The listing builds one solid part. Answer for the finished solid, in the listing's coordinates (mm). A direction names the side the tool comes from. Coordinates: 2 decimals unless noted, no trailing zeros. Order: outer loops, then holes, each group sorted by start corner. A loop starts at its lowest first (then second) coordinate and runs counter-clockwise, first axis right, second up. Notation, with made-up numbers: (78, 13.5) -> (125, 13.5) arc R22 ccw to (125, 26.5) -> close; hole circle Ø4 at (73, 11.25). An arc over 180 degrees is marked (long way). Answer in a Markdown table with one row per item.
```python
from build123d import *

# Parameters (mm, degrees)
F0_R     = 58.419928
F0_R_2   = 50.653175
F4_DEPTH = 8.255


with BuildPart() as f3:
    # F1 (on Right) → F3 (revolve)
    with BuildSketch(Plane.YZ):
        with BuildLine():
            Line((-9.656509, 58.766587), (9.687974, 58.134703))
            ThreePointArc((9.687974, 58.134703), (0.316333, 67.653236), (-9.656509, 58.766587))
        make_face()
    revolve(axis=Axis((0, -0.11386, 0), (0, -1, 0)))

    # F0 (on Front) → F4 (join, symmetric)
    with BuildSketch(Plane.XZ):
        Circle(F0_R)
        Circle(F0_R_2, mode=Mode.SUBTRACT)
    extrude(amount=F4_DEPTH, both=True)


solid = f3.part
```
(1) Find the intervals of material crossed by line 1 along X through (y, z) = (-5, -23); line 2 along Z through (x, y) = (52.5, -4); line 3 along X through (y, z) = (-6, 21.5), in increasing order. Write a range as from..to.
Check values:
| item | result |
|---|---|
| line 1 | -62.15..-53.91, -53.7..-45.13, 45.13..53.7, 53.91..62.15 |
| line 2 | -41.29..-25.99, -25.62..25.62, 25.99..41.29 |
| line 3 | -61.95..-54.56, -54.32..-45.86, 45.86..54.32, 54.56..61.95 |
(2) A cutting plane is placed at C-C, the plane y = 2.5. Determine the outline of the cut face in (x, z), then the cut area to 3 significant figures.
Check values:
| item | result |
|---|---|
| outline | circle Ø134.66 at (0, 0); hole circle Ø101.31 at (0, 0) |
| area | 6,180 mm² |
(3) Flat-ended cylindrical pins translate along their axes: pin 1 (5 mm diameter, centred on x = -50, y = -4.5, fed in from +Z); pin 2 (2 mm diameter, centred on y = -0.5, z = 16, fed in from +X); pin 3 (5 mm diameter, centred on y = 0, z = 45, fed in from +X). Find the tip coordinate at first contact, or state that the pin passes through.
Check values:
| item | result |
|---|---|
| pin 1 | z = 47.06 |
| pin 2 | x = 65.97 |
| pin 3 | x = 52.64 |
(4) Which of the six approach directions +Z, -Z, +X, -X, +Y, -Y give full straight-line access (tool end or side, diameter ignored) to faces 1 (the flat face through (-18, -8.255, 48)), 2 (the cylindrical face through (-50.604, 0.116, 2.227))?
Check values:
| item | result |
|---|---|
| face 1 | -Y |
| face 2 | +Y, -Y |
